For this review, use the dimensioned drawing (mm, ordinates from the lowest corner) and the shaded views. A direction names the side the tool comes from. Give positions to 0.01 mm unless a question says otherwise; leave off trailing zeros. Write each loop counter-clockwise with the first axis right and the second up, starting at its lowest first coordinate (ties: lowest second). Pieces come first, ordered by that corner, then holes. Notation, with made-up numbers: (3.25, 24.25) -> (15.25, 24.25) arc R11 ccw to (15.25, 35.25) -> close; hole circle Ø2 at (81, 21). An arc over 180 degrees is marked (long way). Write each question's results on one line, items separated by ' | '. Start each with the question number.
(1) For the marked faces 1 and 2, list the 3-axis set-ups (+Z, -Z, +X, -X, +Y, -Y) from which the entire face can be reached by the end or side of a thin tool; tool diameter is ignored.
(2) Take a section at A-A (y = 5). State the section outline as (x, z) points.
(3) Take a section at B-B (x = 5). State the section outline as (y, z) points.
(4) To check wall thickness, follow probe 1 along Y at (x, z) = (5, 4.05); probe 2 along X at (y, z) = (4.25, 3.75) (1 decimal); probe 3 along Y at (x, z) = (6, 0.6). State the ranges of each line that lie inside material, in increasing order.
(5) Mouldability with a two-part tool opening along Y and no side actions: class the marked faces 3, 4 and 5 as released by +Y, released by -Y, zero draft, split by the parting line, or undercut.
(6) Clearance check with flat-ended pins moving along their axes: pin 1 (1.5 mm diameter, centred on y = 7, z = 1.5, fed in from -X); pin 2 (1.5 mm diameter, centred on y = 1.5, z = 1.5, fed in from -X) (1 decimal); pin 3 (1 mm diameter, centred on x = 8.5, z = 1, fed in from +Y). State where each tip first meets the part, or that it passes through.
(7) Take a section at C-C (z = 5.05). State the section outline as (x, y) points, plus the area to 3 significant figures.
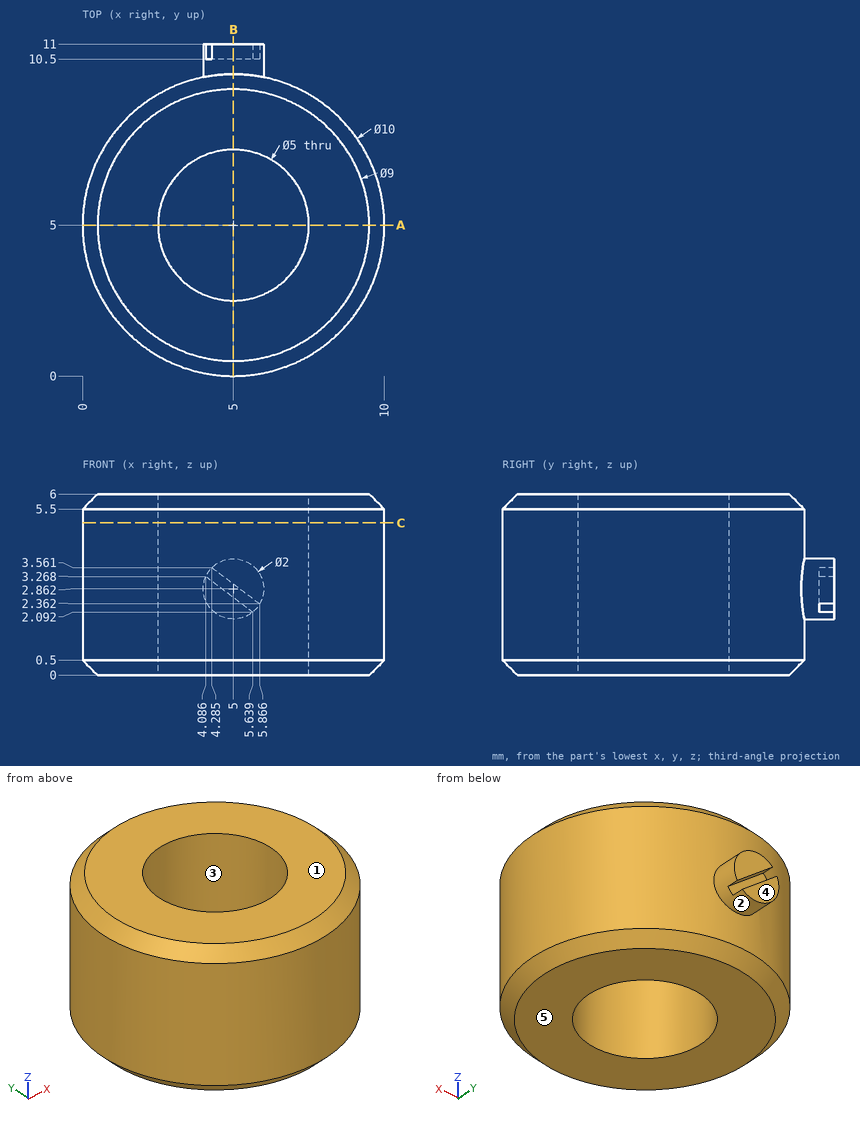
Report:
1) face 1: +Z, +X, -X, +Y, -Y | face 2: +Y
2) outline: (0, 0.5) -> (0.5, 0) -> (2.5, 0) -> (2.5, 6) -> (0.5, 6) -> (0, 5.5) -> close; (7.5, 0) -> (9.5, 0) -> (10, 0.5) -> (10, 5.5) -> (9.5, 6) -> (7.5, 6) -> close
3) outline: (0, 0.5) -> (0.5, 0) -> (2.5, 0) -> (2.5, 6) -> (0.5, 6) -> (0, 5.5) -> close; (7.5, 0) -> (9.5, 0) -> (10, 0.5) -> (10, 1.86) -> (11, 1.86) -> (11, 2.58) -> (10.5, 2.58) -> (10.5, 3.02) -> (11, 3.02) -> (11, 3.86) -> (10, 3.86) -> (10, 5.5) -> (9.5, 6) -> (7.5, 6) -> close
4) probe 1: 0 to 2.5, 7.5 to 10 | probe 2: 0.1 to 2.6, 7.4 to 9.9 | probe 3: 0.1 to 2.71, 7.29 to 9.9
5) face 3: undercut | face 4: released by +Y | face 5: zero draft
6) pin 1: x = 0.16 | pin 2: x = 0.8 | pin 3: y = 9
7) outline: circle Ø10 at (5, 5); hole circle Ø5 at (5, 5) | area: 58.9 mm2
